Answer from the drawing. Dimensions are ordinates in mm from the lowest x, y and z of the part. A direction names the side the tool comes from. Round coordinates to 2 decimals unless told otherwise and drop trailing zeros. Order: outer loops, then holes, each group sorted by start corner. A loop starts at its lowest first (then second) coordinate and runs counter-clockwise, first axis right, second up.
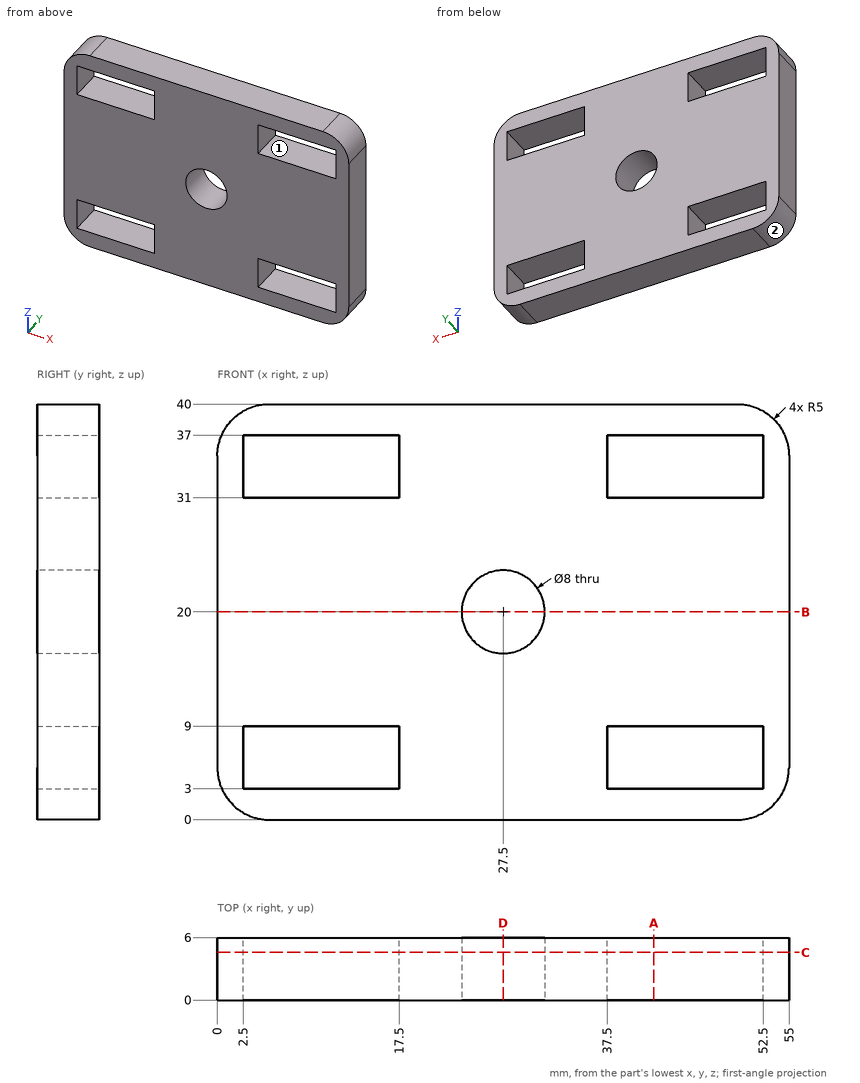
Q1. A cutting plane is placed at C-C, the plane y = 4.6. Give the vertices of the cut face in (x, z).
Outcome:
outline: (0, 5) arc R5 ccw to (5, 0) - (50, 0) arc R5 ccw to (55, 5) - (55, 35) arc R5 ccw to (50, 40) - (5, 40) arc R5 ccw to (0, 35) - close; hole (2.5, 3) - (17.5, 3) - (17.5, 9) - (2.5, 9) - close; hole (2.5, 31) - (17.5, 31) - (17.5, 37) - (2.5, 37) - close; hole circle Ø8 at (27.5, 20); hole (37.5, 3) - (52.5, 3) - (52.5, 9) - (37.5, 9) - close; hole (37.5, 31) - (52.5, 31) - (52.5, 37) - (37.5, 37) - close
Q2. A flat-ended cylindrical pin translates along its axis: pin 1 (7 mm diameter, centred on x = 27.5, z = 20, fed in from -Y). Find the tip coordinate at first contact, or state that the pin passes through.
Outcome:
pin 1: passes through
Q3. A cutting plane is placed at A-A, the plane x = 42. Give the vertices of the cut face in (y, z), plus the area to 3 significant figures.
Outcome:
outline: (0, 0) - (6, 0) - (6, 3) - (0, 3) - close; (0, 9) - (6, 9) - (6, 31) - (0, 31) - close; (0, 37) - (6, 37) - (6, 40) - (0, 40) - close
area: 168 mm2
Q4. A cutting plane is placed at D-D, the plane x = 27.5. Give the vertices of the cut face in (y, z).
Outcome:
outline: (0, 0) - (6, 0) - (6, 16) - (0, 16) - close; (0, 24) - (6, 24) - (6, 40) - (0, 40) - close
Q5. Straight lines are drawn through the part: probe 1 along X at (y, z) = (4.75, 33); probe 2 along Z at (x, y) = (50, 1.15); probe 3 along X at (y, z) = (4.65, 20). For each, find the intervals that lie inside material, in ascending order.
Outcome:
probe 1: x = 0 to 2.5, 17.5 to 37.5, 52.5 to 55
probe 2: z = 0 to 3, 9 to 31, 37 to 40
probe 3: x = 0 to 23.5, 31.5 to 55
Q6. For the marked faces 1 and 2, determine the directions among +Z, -Z, +X, -X, +Y, -Y from which every point of the face is accessible in a straight line to the end or side of a thin tool.
Outcome:
face 1: +Y, -Y
face 2: -Z, -X, +Y, -Y
Q7. A cutting plane is placed at B-B, the plane z = 20. Give the vertices of the cut face in (x, y), plus the area to 3 significant figures.
Outcome:
outline: (0, 0) - (23.5, 0) - (23.5, 6) - (0, 6) - close; (31.5, 0) - (55, 0) - (55, 6) - (31.5, 6) - close
area: 282 mm2
